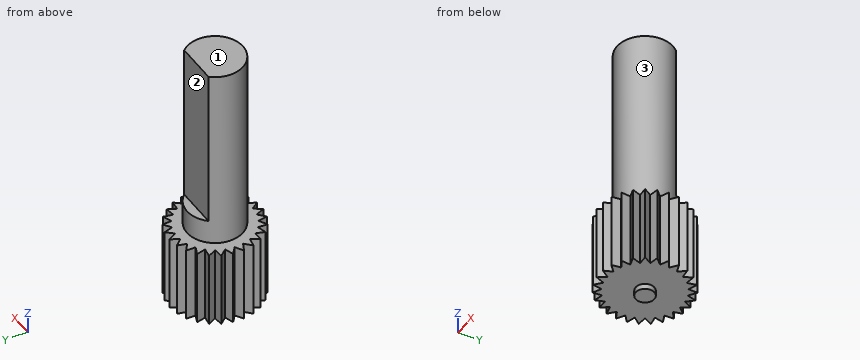
Autodesk Inventor part; units mm, degrees
ref_plane "YZ Plane" through (0, 0, 0) normal (1, 0, 0) x (0, 1, 0)
ref_plane "XZ Plane" through (0, 0, 0) normal (0, 1, 0) x (-1, 0, 0)
ref_plane "XY Plane" through (0, 0, 0) normal (0, 0, 1) x (1, 0, 0)
sketch "Sketch1" plane through (0, 0, 0) normal (0, 0, 1) x (1, 0, 0)
  circle A0 centre (0, 0) radius 0.5
  dimension "d0" = 1
extrude "Extrusion1" add sketch "Sketch1" along normal blind 4.4
sketch "Sketch2" plane through (0, 0, 4.4) normal (0, 0, 1) x (1, 0, 0)
  circle A0 centre (0, 0) radius 0.5
  circle A1 centre (0, 0) radius 2
  dimension "d3" = 4
extrude "Extrusion2" add sketch "Sketch2" against normal blind 4.1
sketch "Sketch4" plane through (0, 0, 4.4) normal (0, 0, 1) x (1, 0, 0)
  circle A0 centre (0, 0) radius 2
  circle A1 centre (0, 0) radius 1.5
  dimension "d6" = 3
extrude "Extrusion3" add sketch "Sketch4" along normal blind 1.3 contours A1
sketch "Sketch5" plane through (0, 0, 5.7) normal (0, 0, 1) x (1, 0, 0)
  circle A0 centre (0, 0) radius 1.5
  circle A1 centre (0, 0) radius 1.5
  line L0 (0, 0) -> (1.0208, 0)
  line L1 (-1.118, 1) -> (1.118, 1)
  line L2 (0, -1.5) -> (1.5, -1.5)
  dimension "d11" = 2.5
extrude "Extrusion5" add sketch "Sketch5" along normal blind 8.67 contours A0 L1 picked at (0, 0.1667)
sketch "Sketch8" plane through (0, 0, 0.3) normal (0, 0, -1) x (-1, 0, 0)
  circle A0 centre (0, 0) radius 0.5
  circle A1 centre (0, 0) radius 2
  line L0 (0, 0) -> (0, 5.155)
  line L1 (0, 2.4402) -> (-0.2438, 1.9851)
  line L2 (0, 2.4402) -> (0.2438, 1.9851)
  arc A2 (0.2438, 1.9851) -> (-0.2438, 1.9851) centre (0, 0) ccw
  line L3 (-0.2438, 1.9851) -> (0, 2.4402)
  line L4 (0, 2.4402) -> (0.2438, 1.9851)
  line L5 (-0.5628, 2.3745) -> (-0.695, 1.8754)
  line L6 (-0.5628, 2.3745) -> (-0.2206, 1.9878)
  arc A3 (-0.2206, 1.9878) -> (-0.695, 1.8754) centre (0, 0) ccw
  line L7 (-1.0952, 2.1807) -> (-1.1087, 1.6645)
  line L8 (-1.0952, 2.1807) -> (-0.6731, 1.8833)
  arc A4 (-0.6731, 1.8833) -> (-1.1087, 1.6645) centre (0, 0) ccw
  line L9 (-1.5686, 1.8693) -> (-1.4627, 1.364)
  line L10 (-1.5686, 1.8693) -> (-1.0893, 1.6774)
  arc A5 (-1.0893, 1.6774) -> (-1.4627, 1.364) centre (0, 0) ccw
  line L11 (-1.9574, 1.4572) -> (-1.7379, 0.9899)
  line L12 (-1.9574, 1.4572) -> (-1.4467, 1.3809)
  arc A6 (-1.4467, 1.3809) -> (-1.7379, 0.9899) centre (0, 0) ccw
  line L13 (-2.2407, 0.9665) -> (-1.9193, 0.5624)
  line L14 (-2.2407, 0.9665) -> (-1.7262, 1.0101)
  arc A7 (-1.7262, 1.0101) -> (-1.9193, 0.5624) centre (0, 0) ccw
  line L15 (-2.4032, 0.4237) -> (-1.9973, 0.1046)
  line L16 (-2.4032, 0.4237) -> (-1.9126, 0.5848)
  arc A8 (-1.9126, 0.5848) -> (-1.9973, 0.1046) centre (0, 0) ccw
  line L17 (-2.4361, -0.1419) -> (-1.9676, -0.3588)
  line L18 (-2.4361, -0.1419) -> (-1.9959, 0.1279)
  arc A9 (-1.9959, 0.1279) -> (-1.9676, -0.3588) centre (0, 0) ccw
  line L19 (-2.3377, -0.6999) -> (-1.8318, -0.8029)
  line L20 (-2.3377, -0.6999) -> (-1.9716, -0.3358)
  arc A10 (-1.9716, -0.3358) -> (-1.8318, -0.8029) centre (0, 0) ccw
  line L21 (-2.1133, -1.2201) -> (-1.5973, -1.2037)
  line L22 (-2.1133, -1.2201) -> (-1.841, -0.7814)
  arc A11 (-1.841, -0.7814) -> (-1.5973, -1.2037) centre (0, 0) ccw
  line L23 (-1.775, -1.6746) -> (-1.2766, -1.5396)
  line L24 (-1.775, -1.6746) -> (-1.6112, -1.1849)
  arc A12 (-1.6112, -1.1849) -> (-1.2766, -1.5396) centre (0, 0) ccw
  line L25 (-1.3409, -2.0388) -> (-0.8872, -1.7925)
  line L26 (-1.3409, -2.0388) -> (-1.2945, -1.5246)
  arc A13 (-1.2945, -1.5246) -> (-0.8872, -1.7925) centre (0, 0) ccw
  line L27 (-0.8346, -2.2931) -> (-0.4499, -1.9487)
  line L28 (-0.8346, -2.2931) -> (-0.908, -1.782)
  arc A14 (-0.908, -1.782) -> (-0.4499, -1.9487) centre (0, 0) ccw
  line L29 (-0.2833, -2.4237) -> (0.0117, -2)
  line L30 (-0.2833, -2.4237) -> (-0.4726, -1.9434)
  arc A15 (-0.4726, -1.9434) -> (0.0117, -2) centre (0, 0) ccw
  line L31 (0.2833, -2.4237) -> (0.4726, -1.9434)
  line L32 (0.2833, -2.4237) -> (-0.0117, -2)
  arc A16 (-0.0117, -2) -> (0.4726, -1.9434) centre (0, 0) ccw
  line L33 (0.8346, -2.2931) -> (0.908, -1.782)
  line L34 (0.8346, -2.2931) -> (0.4499, -1.9487)
  arc A17 (0.4499, -1.9487) -> (0.908, -1.782) centre (0, 0) ccw
  line L35 (1.3409, -2.0388) -> (1.2945, -1.5246)
  line L36 (1.3409, -2.0388) -> (0.8872, -1.7925)
  arc A18 (0.8872, -1.7925) -> (1.2945, -1.5246) centre (0, 0) ccw
  line L37 (1.775, -1.6746) -> (1.6112, -1.1849)
  line L38 (1.775, -1.6746) -> (1.2766, -1.5396)
  arc A19 (1.2766, -1.5396) -> (1.6112, -1.1849) centre (0, 0) ccw
  line L39 (2.1133, -1.2201) -> (1.841, -0.7814)
  line L40 (2.1133, -1.2201) -> (1.5973, -1.2037)
  arc A20 (1.5973, -1.2037) -> (1.841, -0.7814) centre (0, 0) ccw
  line L41 (2.3377, -0.6999) -> (1.9716, -0.3358)
  line L42 (2.3377, -0.6999) -> (1.8318, -0.8029)
  arc A21 (1.8318, -0.8029) -> (1.9716, -0.3358) centre (0, 0) ccw
  line L43 (2.4361, -0.1419) -> (1.9959, 0.1279)
  line L44 (2.4361, -0.1419) -> (1.9676, -0.3588)
  arc A22 (1.9676, -0.3588) -> (1.9959, 0.1279) centre (0, 0) ccw
  line L45 (2.4032, 0.4237) -> (1.9126, 0.5848)
  line L46 (2.4032, 0.4237) -> (1.9973, 0.1046)
  arc A23 (1.9973, 0.1046) -> (1.9126, 0.5848) centre (0, 0) ccw
  line L47 (2.2407, 0.9665) -> (1.7262, 1.0101)
  line L48 (2.2407, 0.9665) -> (1.9193, 0.5624)
  arc A24 (1.9193, 0.5624) -> (1.7262, 1.0101) centre (0, 0) ccw
  line L49 (1.9574, 1.4572) -> (1.4467, 1.3809)
  line L50 (1.9574, 1.4572) -> (1.7379, 0.9899)
  arc A25 (1.7379, 0.9899) -> (1.4467, 1.3809) centre (0, 0) ccw
  line L51 (1.5686, 1.8693) -> (1.0893, 1.6774)
  line L52 (1.5686, 1.8693) -> (1.4627, 1.364)
  arc A26 (1.4627, 1.364) -> (1.0893, 1.6774) centre (0, 0) ccw
  line L53 (1.0952, 2.1807) -> (0.6731, 1.8833)
  line L54 (1.0952, 2.1807) -> (1.1087, 1.6645)
  arc A27 (1.1087, 1.6645) -> (0.6731, 1.8833) centre (0, 0) ccw
  line L55 (0.5628, 2.3745) -> (0.2206, 1.9878)
  line L56 (0.5628, 2.3745) -> (0.695, 1.8754)
  arc A28 (0.695, 1.8754) -> (0.2206, 1.9878) centre (0, 0) ccw
  dimension "d24" = 360
extrude "Extrusion8" add sketch "Sketch8" against normal up to surface (4.1 mm away) contours A1 L6 L1 L0 | L0 L2 L55 A1 | L55 L2 A1 | A1 L1 L6 | L2 L55 L56 L53 A1 | A1 L8 L5 L6 L1 | L53 L56 A1 | A1 L5 L8 | L56 L53 L54 L51 A1 | A1 L10 L7 L8 L5 | L51 L54 A1 | A1 L7 L10 | L54 L51 L52 L49 A1 | A1 L12 L9 L10 L7 | L49 L52 A1 | A1 L9 L12 | L52 L49 L50 L47 A1 | A1 L14 L11 L12 L9 | L47 L50 A1 | A1 L11 L14 | L50 L47 L48 L45 A1 | A1 L16 L13 L14 L11 | L45 L48 A1 | A1 L13 L16 | L48 L45 L46 L43 A1 | A1 L18 L15 L16 L13 | L43 L46 A1 | A1 L15 L18 | L46 L43 L44 L41 A1 | A1 L20 L17 L18 L15 | A1 L17 L20 | L41 L44 A1 | L41 L42 L39 A1 L44 | A1 L22 L19 L20 L17 | A1 L19 L22 | L39 L42 A1 | L39 L40 L37 A1 L42 | A1 L24 L21 L22 L19 | A1 L21 L24 | L37 L40 A1 | L37 L38 L35 A1 L40 | A1 L26 L23 L24 L21 | A1 L23 L26 | L35 L38 A1 | L35 L36 L33 A1 L38 | A1 L28 L25 L26 L23 | A1 L25 L28 | L33 L36 A1 | L33 L34 L31 A1 L36 | A1 L30 L27 L28 L25 | A1 L27 L30 | L31 L34 A1 | L31 L32 L29 A1 L34 | A1 L32 L29 L30 L27 | A1 L29 L32
properties part number "launcher.motor.shaft"
The listing builds one solid part. Answer for the finished solid, in the listing's coordinates (mm). Face numbers are marked on the shaded views. A direction names the side the tool comes from. Give positions to 0.01 mm unless a question says otherwise; leave off trailing zeros. Write each loop counter-clockwise with the first axis right and the second up, starting at its lowest first coordinate (ties: lowest second). Pieces come first, ordered by that corner, then holes.
1) Find the intervals of material crossed by L1, parallel to X at y = -1.9, z = 4; L2, parallel to Z at x = 1.65, y = -1.5; L3, parallel to Z at x = -0.5, y = -1.25, in increasing order.
2) Section A-A (z = 7) is taken. Write down the section's boundary in (x, y), and give its area (3 significant figures).
3) Section B-B (z = 5.5) is taken. Write down the section's boundary in (x, y), and give its area (3 significant figures).
4) Given P1, Ø1.5, axis at x = 0.5, z = 3.5, coming from the +Y side; P2, Ø2, axis at x = -1.5, z = 6, coming from the -Y side; P3, Ø1.1, axis at x = 0, z = 11.5, coming from the +Y side, each flat-ended and moving along its own axis, determine where each tip first touches the part or whether it passes through.
5) A tool of negligible diameter and unlimited length cuts with its end or side. For the marked faces 1, 2 and 3, from which of +Z, -Z, +X, -X, +Y, -Y can it reach the whole face along a straight path? Write none if from no direction.
Response:
1. L1: x = -1.33 to -1.09, -0.89 to 0.89, 1.09 to 1.33
1. L2: z = 0.3 to 4.4
1. L3: z = 0.3 to 14.37
2. outline: (-1.12, 1) arc R1.5 ccw (long way) to (1.12, 1) - close
2. area: 6.29 mm2
3. outline: circle Ø3 at (0, 0)
3. area: 7.07 mm2
4. P1: stops at y = 2.44
4. P2: stops at y = -1.41
4. P3: stops at y = 1
5. face 1: +Z, +X, -X, +Y, -Y
5. face 2: +Z, +X, -X, +Y
5. face 3: +Z
